Geometry check sheet. Reference: the model listing, model coordinates, mm. A direction names the side the tool comes from. Give positions to 0.01 mm unless a question says otherwise; leave off trailing zeros. Write each loop counter-clockwise with the first axis right and the second up, starting at its lowest first coordinate (ties: lowest second). Pieces come first, ordered by that corner, then holes.
(1) Cross-section at C-C (z = 4). Record the boundary of the cut face in (x, y).
(2) Mould release check, pull along X, two halves, no side actions. Record for faces 1 (the flat face through (7, -12, 13)), 2 (the flat face through (10, 11, 26)), 3 (the flat face through (19.123, -19.061, 2.535)): +X half, -X half, draft (parallel to the pull), parting line (faces both ways), or undercut.
(3) Cross-section at D-D (z = 23.25). Record the boundary of the cut face in (x, y), and give its area (3 significant figures).
(4) Tool access check on faces 4 (the flat face through (-16.901, 23, 3)), 5 (the flat face through (12, -12, 13)), 6 (the flat face through (-11, -9, 16)), 7 (the flat face through (16.901, 23, 3)). Record the directions out of +Z, -Z, +X, -X, +Y, -Y that give a thin tool (end or side, any length) a straight path to the whole face; none if there is none.
(5) Cross-section at B-B (x = -8). Record the boundary of the cut face in (y, z).
(6) Depth check by flat-ended pin: P1, Ø1, axis at x = -11.5, z = 16.5, coming from the +Y side; P2, Ø12, axis at y = -8, z = 19.5, coming from the +X side; P3, Ø6.5, axis at y = 13, z = 17, coming from the -X side; P4, Ø6, axis at y = -17, z = 22.5, coming from the +X side. Enter the tip coordinate at first touch or a pass-through.
(7) Thickness scan on line 1 along Y through (x, z) = (0, 2.4); line 2 along Z through (x, y) = (-20.5, 0.5); line 3 along X through (y, z) = (11.5, 22.5). Record the ranges inside material, lowest first.
(8) Cross-section at A-A (y = 0). Record the boundary of the cut face in (x, z), and give its area (3 significant figures).
Autodesk Inventor part; units mm, degrees
ref_plane "YZ Plane" through (0, 0, 0) normal (1, 0, 0) x (0, 1, 0)
ref_plane "XZ Plane" through (0, 0, 0) normal (0, 1, 0) x (-1, 0, 0)
ref_plane "XY Plane" through (0, 0, 0) normal (0, 0, 1) x (1, 0, 0)
sketch "Sketch1" plane through (0, 0, 0) normal (0, 0, 1) x (1, 0, 0)
  line L0 (-34.86, 0) -> (34.86, 0) construction
  line L1 (0, -34.86) -> (0, 34.86) construction
  line L2 (0, 0) -> (16.9726, 16.9726) construction
  line L3 (0, 0) -> (24.0028, 0) construction
  line L4 (0, 24.9) -> (16.8009, 24.9)
  line L5 (16.8009, 24.9) -> (16.8009, 21.2415)
  line L6 (16.8009, 21.2415) -> (19.0212, 19.0212)
  line L7 (24.9, 0) -> (24.9, 16.8009)
  line L8 (24.9, 16.8009) -> (21.2415, 16.8009)
  line L9 (21.2415, 16.8009) -> (19.0212, 19.0212)
  line L10 (0, -24.9) -> (16.8009, -24.9)
  line L11 (16.8009, -24.9) -> (16.8009, -21.2415)
  line L12 (16.8009, -21.2415) -> (19.0212, -19.0212)
  line L13 (24.9, 0) -> (24.9, -16.8009)
  line L14 (24.9, -16.8009) -> (21.2415, -16.8009)
  line L15 (21.2415, -16.8009) -> (19.0212, -19.0212)
  line L16 (0, 0) -> (-16.9726, 16.9726) construction
  line L17 (0, 0) -> (-24.0028, 0) construction
  line L18 (0, 24.9) -> (-16.8009, 24.9)
  line L19 (-16.8009, 24.9) -> (-16.8009, 21.2415)
  line L20 (-16.8009, 21.2415) -> (-19.0212, 19.0212)
  line L21 (-24.9, 0) -> (-24.9, 16.8009)
  line L22 (-24.9, 16.8009) -> (-21.2415, 16.8009)
  line L23 (-21.2415, 16.8009) -> (-19.0212, 19.0212)
  line L24 (0, -24.9) -> (-16.8009, -24.9)
  line L25 (-16.8009, -24.9) -> (-16.8009, -21.2415)
  line L26 (-16.8009, -21.2415) -> (-19.0212, -19.0212)
  line L27 (-21.2415, -16.8009) -> (-19.0212, -19.0212)
  line L28 (-24.9, -16.8009) -> (-21.2415, -16.8009)
  line L29 (-24.9, 0) -> (-24.9, -16.8009)
  circle A0 centre (0, 0) radius 10
  dimension "d17" = 45
  dimension "d18" = 24.9
  dimension "d20" = 3.14
  dimension "d21" = 26.9
  dimension "d22" = 20
extrude "Extrusion1" add sketch "Sketch1" along normal blind 5
sketch "Sketch2" plane through (0, 0, 5) normal (0, 0, 1) x (1, 0, 0)
  circle A0 centre (0, 0) radius 10
  line L0 (16.8009, 24.9) -> (-16.8009, 24.9)
  line L1 (-16.8009, 24.9) -> (-16.8009, 21.2415)
  line L2 (-16.8009, 21.2415) -> (-21.2415, 16.8009)
  line L3 (-21.2415, 16.8009) -> (-24.9, 16.8009)
  line L4 (-24.9, 16.8009) -> (-24.9, -16.8009)
  line L5 (-24.9, -16.8009) -> (-21.2415, -16.8009)
  line L6 (-21.2415, -16.8009) -> (-16.8009, -21.2415)
  line L7 (-16.8009, -21.2415) -> (-16.8009, -24.9)
  line L8 (-16.8009, -24.9) -> (16.8009, -24.9)
  line L9 (16.8009, -24.9) -> (16.8009, -21.2415)
  line L10 (16.8009, -21.2415) -> (21.2415, -16.8009)
  line L11 (21.2415, -16.8009) -> (24.9, -16.8009)
  line L12 (24.9, -16.8009) -> (24.9, 16.8009)
  line L13 (24.9, 16.8009) -> (21.2415, 16.8009)
  line L14 (21.2415, 16.8009) -> (16.8009, 21.2415)
  line L15 (16.8009, 21.2415) -> (16.8009, 24.9)
  line L16 (0, -34.86) -> (0, 34.86) construction
  line L17 (-12, 12) -> (-7, 12)
  line L18 (-7, 12) -> (-7, 10)
  line L19 (-7, 10) -> (-12, 10)
  line L20 (-12, 10) -> (-12, 12)
  dimension "d27" = 2
  dimension "d28" = 5
  dimension "d29" = 12
extrude "Extrusion2" add sketch "Sketch2" along normal blind 21 contours L17 L18 L19 L20
sketch "Sketch4" plane through (-12, 10, 5) normal (-1, 0, 0) x (0, 0, 1)
  line L0 (0, 0) -> (0, 2)
  line L1 (0, 0) -> (21, 0)
  line L2 (21, 2) -> (21, 0)
  line L3 (0, 2) -> (21, 2)
  line L4 (0, 6.8009) -> (0, -26.8009)
  line L5 (0, 2) -> (21, 2)
  line L6 (21, 2) -> (0, 2)
  line L7 (0, 2) -> (0, 6)
  line L8 (0, -26.8009) -> (0, 6.8009)
  line L9 (0, 6) -> (21, 2)
  point P0 (-5, -10)
  dimension "d35" = 4
extrude "Extrusion4" add sketch "Sketch4" against normal up to surface (5 mm away) contours L4 L9 L3
sketch "Sketch5" plane through (-12, 10, 5) normal (0, -1, 0) x (1, 0, 0)
  line L0 (5, 21) -> (5, 0)
  line L1 (0, 0) -> (5, 0)
  line L2 (0, 21) -> (0, 0)
  line L3 (5, 21) -> (0, 21)
  line L4 (12, -10.2) -> (12, 26.2) construction
  line L5 (0, 21) -> (2, 21)
  line L6 (2, 21) -> (2, 0)
  line L7 (2, 0) -> (0, 0)
  line L8 (0, 0) -> (0, 21)
  point P0 (12, -5)
  dimension "d38" = 10
extrude "Extrusion5" add sketch "Sketch5" along normal blind 1 contours L6 L1 L2 L3
mirror "Mirror1" about plane through (0, 0, 0) normal (0, 1, 0) of "Extrusion2", "Extrusion4", "Extrusion5"
mirror "Mirror2" about plane through (0, 0, 0) normal (1, 0, 0) of "Extrusion2", "Extrusion4", "Mirror1", "Extrusion5"
sketch "Skizze6" plane through (0, 0, 5) normal (0, 0, 1) x (1, 0, 0)
  line L0 (12, -16) -> (7, -16) construction
  line L1 (7, -16) -> (7, -10) construction
  line L2 (7, -10) -> (10, -10) construction
  line L3 (10, -10) -> (10, -9) construction
  line L4 (10, -9) -> (12, -9) construction
  line L5 (12, -9) -> (12, -16) construction
  line L6 (7, 16) -> (12, 16) construction
  line L7 (12, 16) -> (12, 9) construction
  line L8 (12, 9) -> (10, 9) construction
  line L9 (10, 9) -> (10, 10) construction
  line L10 (10, 10) -> (7, 10) construction
  line L11 (7, 10) -> (7, 16) construction
  line L12 (-7, -16) -> (-12, -16) construction
  line L13 (-12, -16) -> (-12, -9) construction
  line L14 (-12, -9) -> (-10, -9) construction
  line L15 (-10, -9) -> (-10, -10) construction
  line L16 (-10, -10) -> (-7, -10) construction
  line L17 (-7, -10) -> (-7, -16) construction
  line L18 (-12, 9) -> (-12, 16) construction
  line L19 (-12, 16) -> (-7, 16) construction
  line L20 (-7, 16) -> (-7, 10) construction
  line L21 (-7, 10) -> (-10, 10) construction
  line L22 (-10, 10) -> (-10, 9) construction
  line L23 (-10, 9) -> (-12, 9) construction
  circle A0 centre (0, 0) radius 10 construction
  line L24 (16.8009, 24.9) -> (-16.8009, 24.9) construction
  line L25 (-16.8009, 24.9) -> (-16.8009, 21.2415)
  line L26 (-16.8009, 21.2415) -> (-21.2415, 16.8009)
  line L27 (-21.2415, 16.8009) -> (-24.9, 16.8009)
  line L28 (-24.9, 16.8009) -> (-24.9, -16.8009) construction
  line L29 (-24.9, -16.8009) -> (-21.2415, -16.8009)
  line L30 (-21.2415, -16.8009) -> (-16.8009, -21.2415)
  line L31 (-16.8009, -21.2415) -> (-16.8009, -24.9)
  line L32 (-16.8009, -24.9) -> (16.8009, -24.9) construction
  line L33 (16.8009, -24.9) -> (16.8009, -21.2415)
  line L34 (16.8009, -21.2415) -> (21.2415, -16.8009)
  line L35 (21.2415, -16.8009) -> (24.9, -16.8009)
  line L36 (24.9, -16.8009) -> (24.9, 16.8009) construction
  line L37 (24.9, 16.8009) -> (21.2415, 16.8009)
  line L38 (21.2415, 16.8009) -> (16.8009, 21.2415)
  line L39 (16.8009, 21.2415) -> (16.8009, 24.9)
  line L40 (-16.9009, 25) -> (16.9009, 25) construction
  line L41 (16.9009, 25) -> (16.9009, 21.2829)
  line L42 (16.9009, 21.2829) -> (21.2829, 16.9009)
  line L43 (21.2829, 16.9009) -> (25, 16.9009)
  line L44 (25, 16.9009) -> (25, -16.9009) construction
  line L45 (25, -16.9009) -> (21.2829, -16.9009)
  line L46 (21.2829, -16.9009) -> (16.9009, -21.2829)
  line L47 (16.9009, -21.2829) -> (16.9009, -25)
  line L48 (16.9009, -25) -> (-16.9009, -25) construction
  line L49 (-16.9009, -25) -> (-16.9009, -21.2829)
  line L50 (-16.9009, -21.2829) -> (-21.2829, -16.9009)
  line L51 (-21.2829, -16.9009) -> (-25, -16.9009)
  line L52 (-25, -16.9009) -> (-25, 16.9009) construction
  line L53 (-25, 16.9009) -> (-21.2829, 16.9009)
  line L54 (-21.2829, 16.9009) -> (-16.9009, 21.2829)
  line L55 (-16.9009, 21.2829) -> (-16.9009, 25)
  line L56 (-24.9, 16.8009) -> (-24.9, 16.9009)
  line L57 (-16.8009, 24.9) -> (-16.9009, 24.9)
  line L58 (16.8009, 24.9) -> (-16.8009, 24.9)
  line L59 (16.8009, 24.9) -> (16.9009, 24.9)
  line L60 (24.9, 16.8009) -> (24.9, 16.9009)
  line L61 (16.8009, -24.9) -> (16.9009, -24.9)
  line L62 (21.2415, -16.8009) -> (24.9, -16.8009)
  line L63 (24.9, -16.8009) -> (24.9, -16.9009)
  line L64 (-16.8009, -24.9) -> (-16.9009, -24.9)
  line L65 (-24.9, -16.8009) -> (-21.2415, -16.8009)
  line L66 (-24.9, -16.8009) -> (-24.9, -16.9009)
  dimension "d17" = 45
  dimension "d18" = 24.9
  dimension "d20" = 3.14
  dimension "d21" = 26.9
  dimension "d41" = 0.1
extrude "IM_offset" add sketch "Skizze6" against normal up to surface (5 mm away)
properties part number "20_Cube_Insert_Beamsplitter_v3"
Reply:
1. outline: (-24.9, -16.9) - (-21.28, -16.9) - (-16.9, -21.28) - (-16.9, -24.9) - (16.9, -24.9) - (16.9, -21.28) - (21.28, -16.9) - (24.9, -16.9) - (24.9, 16.9) - (21.28, 16.9) - (16.9, 21.28) - (16.9, 24.9) - (-16.9, 24.9) - (-16.9, 21.28) - (-21.28, 16.9) - (-24.9, 16.9) - close; hole circle Ø20 at (0, 0)
2. face 1: undercut
2. face 2: draft
2. face 3: +X half
3. outline: (-12, -12.52) - (-7, -12.52) - (-7, -10) - (-10, -10) - (-10, -9) - (-12, -9) - close; (-12, 9) - (-10, 9) - (-10, 10) - (-7, 10) - (-7, 12.52) - (-12, 12.52) - close; (7, -12.52) - (12, -12.52) - (12, -9) - (10, -9) - (10, -10) - (7, -10) - close; (7, 10) - (10, 10) - (10, 9) - (12, 9) - (12, 12.52) - (7, 12.52) - close
3. area: 58.5 mm2
4. face 4: +Z, -Z, -X, +Y
4. face 5: +Z, +X, +Y, -Y
4. face 6: +Z, +X, -X
4. face 7: +Z, -Z, +X, +Y
5. outline: (-24.9, 0) - (-6, 0) - (-6, 5) - (-10, 5) - (-10, 26) - (-12, 26) - (-16, 5) - (-24.9, 5) - close; (6, 0) - (24.9, 0) - (24.9, 5) - (16, 5) - (12, 26) - (10, 26) - (10, 5) - (6, 5) - close
6. P1: stops at y = 13.9
6. P2: stops at x = 12
6. P3: stops at x = -12
6. P4: passes through
7. line 1: y = -24.9 to -10, 10 to 24.9
7. line 2: z = 0 to 5
7. line 3: x = -12 to -7, 7 to 12
8. outline: (-24.9, 0) - (-10, 0) - (-10, 5) - (-24.9, 5) - close; (10, 0) - (24.9, 0) - (24.9, 5) - (10, 5) - close
8. area: 149 mm2
